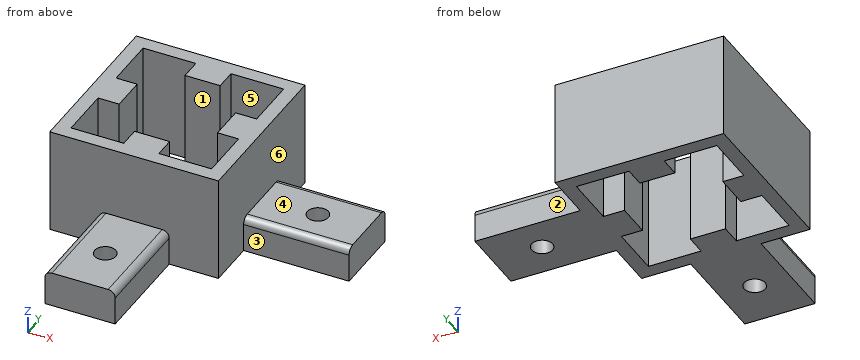
```python
from build123d import *

# Parameters (mm, degrees)
SKETCH2_W           = 24
SKETCH2_H           = 24
BOSS_EXTRUDE1_DEPTH = 15
BOSS_EXTRUDE2_DEPTH = 15
CUT_EXTRUDE1_REACH  = 33.193
SKETCH4_R           = 1.5
CIRPATTERN1_COUNT   = 2
CIRPATTERN1_ANGLE   = 90


with BuildPart() as part:
    # Sketch2 → Boss-Extrude1 (new body)
    with BuildSketch(Plane.XY):
        Rectangle(SKETCH2_W, SKETCH2_H)
        Polygon((-2.5, 10), (-2.5, 7), (2.5, 7), (2.5, 10), (10, 10), (10, 2.5), (7, 2.5), (7, -2.5), (10, -2.5), (10, -10), (2.5, -10), (2.5, -7), (-2.5, -7), (-2.5, -10), (-10, -10), (-10, -2.5), (-7, -2.5), (-7, 2.5), (-10, 2.5), (-10, 10), align=None, mode=Mode.SUBTRACT)
    extrude(amount=BOSS_EXTRUDE1_DEPTH)

    # Sketch3 → Boss-Extrude2 (add)
    with BuildSketch(Plane.XZ.offset(12)):
        with BuildLine():
            Line((-5, 4), (-5, 0))
            Line((-5, 0), (5, 0))
            Line((5, 0), (5, 4))
            ThreePointArc((5, 4), (4.707106781, 4.707106781), (4, 5))
            Line((4, 5), (-4, 5))
            ThreePointArc((-4, 5), (-4.707106781, 4.707106781), (-5, 4))
        make_face()
    boss_extrude2 = extrude(amount=BOSS_EXTRUDE2_DEPTH)

    # Sketch4 → Cut-Extrude1 (cut, up to next)
    with BuildSketch(Plane.XY.offset(5), mode=Mode.PRIVATE) as cut_extrude1_sk1:
        with Locations((0, -20)):
            Circle(SKETCH4_R)
    cut_extrude1_tool1 = extrude(cut_extrude1_sk1.sketch, amount=-CUT_EXTRUDE1_REACH, mode=Mode.PRIVATE) & part.part
    cut_extrude1 = cut_extrude1_tool1.solids().sort_by_distance((0, -20, 5))[0]
    add(cut_extrude1, mode=Mode.SUBTRACT)

    # CirPattern1: Boss-Extrude2, Cut-Extrude1 ×2 about axis
    cirpattern1_axis = Axis((0, 0, 0), (0, 0, 1))
    add([boss_extrude2.rotate(cirpattern1_axis, i * CIRPATTERN1_ANGLE / (CIRPATTERN1_COUNT - 1)) for i in range(1, CIRPATTERN1_COUNT)])
    add([cut_extrude1.rotate(cirpattern1_axis, i * CIRPATTERN1_ANGLE / (CIRPATTERN1_COUNT - 1)) for i in range(1, CIRPATTERN1_COUNT)], mode=Mode.SUBTRACT)


solid = part.part
```
For this review, take the finished solid that the model builds, in its own axes (mm). Face numbers are marked on the shaded views. A direction names the side the tool comes from. Coordinates: 2 decimals unless noted, no trailing zeros. Order: outer loops, then holes, each group sorted by start corner. A loop starts at its lowest first (then second) coordinate and runs counter-clockwise, first axis right, second up. Notation, with made-up numbers: (-32, 37.25) - (-23, 37.25) arc R11 cw to (-23, 50.25) - close; hole circle Ø2 at (-36.75, 34.25). An arc over 180 degrees is marked (long way). Answer as a JSON object with one key per item and string values. Group by question number.
1. We need section C-C on z = 1.5. Give the number of separate pieces and of enclosed holes in the cut face, then the cut area to 3 significant figures.
2. We need section D-D on y = 0. State the section outline as (x, z) points.
3. For probe 1 along Y at (x, z) = (8.5, 12.25); probe 2 along X at (y, z) = (0, 4.05); probe 3 along Y at (x, z) = (0, 2.15), list the stretches that pass through material, from the lowest coordinate up.
4. For the marked faces 1, 2 and 3, list the 3-axis set-ups (+Z, -Z, +X, -X, +Y, -Y) from which the entire face can be reached by the end or side of a thin tool; tool diameter is ignored.
5. We need section A-A on y = -20. State the section outline as (x, z) points.
6. Clearance check with flat-ended pins moving along their axes: P1, Ø2, axis at x = 20, z = 5.5, coming from the +Y side; P2, Ø3.5, axis at y = -8, z = 7, coming from the +X side; P3, Ø3, axis at x = 18.5, z = 2, coming from the +Y side. State where each tip first meets the part, or that it passes through.
7. The part is to be moulded in two halves that separate along X. For the marked faces 4, 5 and 6, say which applies: pulls with the +X half, pulls with the -X half, needs draft (parallel to the pull), parting line crosses it, or undercut.
Final values:
{
 "1": {"separate pieces": "1", "enclosed holes": "3", "area": "522 mm²"},
 "2": {"outline": "(-12, 0) - (-7, 0) - (-7, 15) - (-12, 15) - close; (7, 0) - (18.5, 0) - (18.5, 5) - (12, 5) - (12, 15) - (7, 15) - close; (21.5, 0) - (27, 0) - (27, 5) - (21.5, 5) - close"},
 "3": {"probe 1": "-12 to -10, -2.5 to 2.5, 10 to 12", "probe 2": "-12 to -7, 7 to 18.5, 21.5 to 27", "probe 3": "-27 to -21.5, -18.5 to -7, 7 to 12"},
 "4": {"face 1": "+Z, -Z", "face 2": "+Z, -Z, +X, +Y", "face 3": "+Z, -Z, +X, -Y"},
 "5": {"outline": "(-5, 0) - (-1.5, 0) - (-1.5, 5) - (-4, 5) arc R1 ccw to (-5, 4) - close; (1.5, 0) - (5, 0) - (5, 4) arc R1 ccw to (4, 5) - (1.5, 5) - close"},
 "6": {"P1": "y = 4.87", "P2": "x = 12", "P3": "y = 5"},
 "7": {"face 4": "needs draft", "face 5": "undercut", "face 6": "pulls with the +X half"}
}
